Source: CAD feature listing. Evaluate the final solid. Frame: model axes, mm. Face numbers are marked on the shaded views. A direction names the side the tool comes from. Coordinates: 2 decimals unless noted, no trailing zeros. Write each loop counter-clockwise with the first axis right and the second up, starting at its lowest first coordinate (ties: lowest second). Pieces come first, ordered by that corner, then holes. Notation, with made-up numbers: M 85.5,60 L 134.5,60 A20 ccw 134.5,76 Z; hole C -14,86.5 d1. An arc over 180 degrees is marked long. One line per item, written item: value. Start each with the question number.
Item 1: Pin query (flat end, axial travel): P1, Ø18.5, axis at x = 11, y = -50, coming from the +Z side; P2, Ø15, axis at y = -28.5, z = 47, coming from the +X side; P3, Ø13, axis at x = 26.5, y = -62.5, coming from the +Z side; P4, Ø5, axis at x = 91.5, z = 44, coming from the +Y side. Return the tip coordinate at first contact, or that it passes through.
Item 2: Set-up query: the marked faces 4, 5 and 6. Return all of +Z, -Z, +X, -X, +Y, -Y with unobstructed straight access to the full face (end or side cutting, diameter ignored); none if empty.
Item 3: Mould query, pull axis X, two halves, no side actions, for the marked faces 1, 2 and 3. Classes: released by +X, released by -X, zero draft, split by the parting line, or undercut.
Item 4: Cut plane D-D, the plane z = 12. Output: boundary loops of the cut face in (x, y), then the cut area to 3 significant figures.
Item 5: Cut plane A-A, the plane x = 96. Output: boundary loops of the cut face in (y, z).
Item 6: Cut plane C-C, the plane z = 24. Output: boundary loops of the cut face in (x, y).
Item 7: Cut plane B-B, the plane y = -58. Output: boundary loops of the cut face in (x, z), then the cut area to 3 significant figures.
Item 8: Ray query, L1, parallel to Y at x = 75, z = 4.5; L2, parallel to X at y = -59.5, z = 26; L3, parallel to X at y = -54, z = 33. Return the intervals inside material, ascending. Write a range as from..to.
```python
from build123d import *

# Parameters (mm, degrees)
SKETCH_2_W          = 23
SKETCH_2_H          = 83.54692924
EXTRUDE_1_DEPTH     = 20
SKETCH_2_W_2        = 115
SKETCH_2_R          = 22.5
EXTRUDE_1_2_DEPTH   = 20
SKETCH_2_3_W        = 12
SKETCH_2_3_H        = 83.54692924
EXTRUDE_2_DEPTH     = 30
SKETCH_4_W          = 13.50460444
SKETCH_4_H          = 50.449539632
EXTRUDE_4_DEPTH     = 83.54692924
SKETCH_6_R          = 12.5
CUT_EXTRUDE_1_DEPTH = 164.164371188
EXTRUDE_5_DEPTH     = 10


with BuildPart() as part:
    # Sketch 2 → Extrude 1 (new body)
    with BuildSketch(Plane.XY):
        with Locations((11.5, -41.77346462)):
            Rectangle(SKETCH_2_W, SKETCH_2_H)
    extrude(amount=EXTRUDE_1_DEPTH)



with BuildPart() as body_2:
    # Sketch 2 → Extrude 1 2 (new body)
    with BuildSketch(Plane.XY):
        with Locations((92.5, -41.77346462)):
            Rectangle(SKETCH_2_W_2, SKETCH_2_H)
        with Locations((75, -41.77346462)):
            Circle(SKETCH_2_R, mode=Mode.SUBTRACT)
    extrude(amount=EXTRUDE_1_2_DEPTH)


with BuildPart() as part_1:
    add(part.part)

    add(body_2.part)  # Extrude 2 merges body 2
    # Sketch 2_3 → Extrude 2 (add)
    with BuildSketch(Plane.XY):
        with Locations((29, -41.77346462)):
            Rectangle(SKETCH_2_3_W, SKETCH_2_3_H)
    extrude(amount=EXTRUDE_2_DEPTH)

    # Sketch 4 → Extrude 4 (add)
    with BuildSketch(Plane(origin=(0, 0, 0), x_dir=(1, 0, 0), z_dir=(0, 1, 0))):
        with Locations((127.910814118, -45.224769816)):
            Rectangle(SKETCH_4_W, SKETCH_4_H)
    extrude(amount=-EXTRUDE_4_DEPTH)

    # Sketch 6 → Cut-Extrude 1 (cut, through all)
    with BuildSketch(Plane.ZY.offset(-121.158511898)):
        with Locations((45.224769816, -41.77346462)):
            Circle(SKETCH_6_R)
    extrude(amount=-CUT_EXTRUDE_1_DEPTH, mode=Mode.SUBTRACT)

    # Sketch 7 → Extrude 5 (add)
    with BuildSketch(Plane(origin=(0, 0, 0), x_dir=(1, 0, 0), z_dir=(0, 1, 0))):
        Polygon((121.158511898, -70.449539632), (70.320934242, -20), (121.158511898, -20), align=None)
    extrude(amount=-EXTRUDE_5_DEPTH)


solid = part_1.part
```
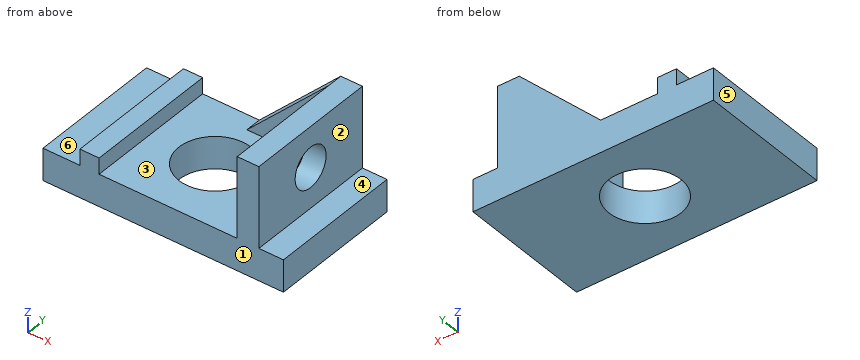
From the geometry:
1. P1: stops at z = 20
1. P2: stops at x = 134.66
1. P3: stops at z = 30
1. P4: stops at y = 0
2. face 4: +Z, +X, +Y, -Y
2. face 5: +Z, -Z, -X, +Y, -Y
2. face 6: +Z, -X, +Y, -Y
3. face 1: zero draft
3. face 2: released by +X
3. face 3: undercut
4. outline: M 0,-83.55 L 150,-83.55 L 150,0 L 0,0 Z; hole C 75,-41.77 d45
4. area: 10,900 mm²
5. outline: M -83.55,0 L -49.85,0 L -49.85,20 L -83.55,20 Z; M -33.7,0 L 0,0 L 0,45.48 L -10,45.48 L -10,20 L -33.7,20 Z
6. outline: M 23,-83.55 L 35,-83.55 L 35,0 L 23,0 Z; M 74.35,-10 L 121.16,-10 L 121.16,-83.55 L 134.66,-83.55 L 134.66,0 L 74.35,0 Z
7. outline: M 0,0 L 59.41,0 L 59.41,20 L 35,20 L 35,30 L 23,30 L 23,20 L 0,20 Z; M 90.59,0 L 150,0 L 150,20 L 134.66,20 L 134.66,70.45 L 121.16,70.45 L 121.16,20 L 90.59,20 Z
7. area: 3,180 mm²
8. L1: y = -83.55..-64.27, -19.27..0
8. L2: x = 23..35, 121.16..134.66
8. L3: x = 121.16..134.66
